from build123d import *
from build123d.topology import SkipClean

# Parameters (mm, degrees)
SKETCH2_R           = 2.5
BOSS_EXTRUDE1_DEPTH = 7
FILLET1_R           = 90
BOSS_EXTRUDE3_DEPTH = 15
SKETCH4_R           = 8
CUT_EXTRUDE1_DEPTH  = 10
BOSS_EXTRUDE4_START = 10
BOSS_EXTRUDE4_DEPTH = 10


with BuildPart() as part:
    # Sketch2 → Boss-Extrude1 (new body)
    with BuildSketch(Plane(origin=(0, 0, 0), x_dir=(1, 0, 0), z_dir=(0, 1, 0))):
        with BuildLine():
            Line((-4.24846021, -9.602113613), (13.572308451, -17.486922065))
            ThreePointArc((13.572308451, -17.486922065), (20.638500285, -15.805826469), (20.907079545, -8.547382103))
            Line((20.907079545, -8.547382103), (11.451696022, 4.891208687))
            ThreePointArc((11.451696022, 4.891208687), (9.270724445, 7.034926316), (6.472222222, 8.268031175))
            ThreePointArc((6.472222222, 8.268031175), (4.86754966, 9.30359932), (3.101845071, 10.031378627))
            Line((3.101845071, 10.031378627), (-8.821699821, 13.718308443))
            ThreePointArc((-8.821699821, 13.718308443), (-15.091857172, 11.987583677), (-16.147811194, 5.569231667))
            Line((-16.147811194, 5.569231667), (-12.308520784, -3.358124948))
            ThreePointArc((-12.308520784, -3.358124948), (-9.971976629, -6.504419403), (-6.472222222, -8.268031175))
            ThreePointArc((-6.472222222, -8.268031175), (-5.401685102, -9.003987898), (-4.24846021, -9.602113613))
        make_face()
        with Locations(Location((16, -12, 0), (0, 0, 270))):
            Circle(SKETCH2_R, mode=Mode.SUBTRACT)
        with Locations(Location((-10.604337088, 7.953252816, 0), (0, 0, 270))):
            Circle(SKETCH2_R, mode=Mode.SUBTRACT)
        with BuildLine():
            ThreePointArc((-4.694444444, -4.495797077), (0, -6.5), (4.694444444, -4.495797077))
            ThreePointArc((4.694444444, -4.495797077), (9, 0), (4.694444444, 4.495797077))
            ThreePointArc((4.694444444, 4.495797077), (0, 6.5), (-4.694444444, 4.495797077))
            ThreePointArc((-4.694444444, 4.495797077), (-9, 0), (-4.694444444, -4.495797077))
        make_face(mode=Mode.SUBTRACT)
    extrude(amount=BOSS_EXTRUDE1_DEPTH)

    # Fillet1
    fillet1_edges = [part.edges().sort_by_distance(p)[0] for p in [
        (6.472222222, 3.5, -8.268031175),
        (-6.472222222, 3.5, 8.268031175),
    ]]
    fillet(fillet1_edges, radius=FILLET1_R)

    # Sketch3 → Boss-Extrude3 (add)
    with BuildSketch(Plane(origin=(0, 7, 0), x_dir=(1, 0, 0), z_dir=(0, 1, 0))):
        with BuildLine():
            Line((-13.446880098, 1.012795393), (-12.308520784, -3.358124948))
            ThreePointArc((-12.308520784, -3.358124948), (-10.611843956, -5.907229762), (-8.121968415, -7.689690813))
            ThreePointArc((-8.121968415, -7.689690813), (-6.480430757, -8.483296944), (-4.855306799, -9.309994408))
            ThreePointArc((-4.855306799, -9.309994408), (-4.554226262, -9.460920841), (-4.24846021, -9.602113613))
            Line((-4.24846021, -9.602113613), (-1.454246479, -10.838414946))
            ThreePointArc((-1.454246479, -10.838414946), (10.979115699, -7.880432641), (11.451696022, 4.891208687))
            ThreePointArc((11.451696022, 4.891208687), (9.968863726, 6.507036925), (8.121968415, 7.689690813))
            ThreePointArc((8.121968415, 7.689690813), (6.480430757, 8.483296944), (4.855306799, 9.309994408))
            ThreePointArc((4.855306799, 9.309994408), (3.994892398, 9.710346787), (3.101845071, 10.031378627))
            Line((3.101845071, 10.031378627), (-3.895223267, 11.305534387))
            ThreePointArc((-3.895223267, 11.305534387), (-5.691953988, 10.727471116), (-6.207623157, 8.911848981))
            ThreePointArc((-6.207623157, 8.911848981), (-7.30582589, 4.892236012), (-11.232333003, 3.497288147))
            ThreePointArc((-11.232333003, 3.497288147), (-13.004436636, 2.847636589), (-13.446880098, 1.012795393))
        make_face()
        with BuildLine():
            ThreePointArc((4.694444444, -4.495797077), (9, 0), (4.694444444, 4.495797077))
            ThreePointArc((4.694444444, 4.495797077), (0, 6.5), (-4.694444444, 4.495797077))
            ThreePointArc((-4.694444444, 4.495797077), (-9, 0), (-4.694444444, -4.495797077))
            ThreePointArc((-4.694444444, -4.495797077), (0, -6.5), (4.694444444, -4.495797077))
        make_face(mode=Mode.SUBTRACT)
    extrude(amount=BOSS_EXTRUDE3_DEPTH)

    # Sketch4 → Cut-Extrude1 (cut)
    with BuildSketch(Plane(origin=(0, 22, 0), x_dir=(1, 0, 0), z_dir=(0, 1, 0))):
        Circle(SKETCH4_R)
    extrude(amount=-CUT_EXTRUDE1_DEPTH, mode=Mode.SUBTRACT)

    # Sketch5 → Boss-Extrude4 (add)
    with SkipClean():  # the faces are left unmerged after this step: merging them gives an invalid solid
        with BuildSketch(Plane(origin=(0, 12, 0), x_dir=(1, 0, 0), z_dir=(0, 1, 0)).offset(BOSS_EXTRUDE4_START)):
            with BuildLine():
                ThreePointArc((-7.111111111, 3.664982778), (-8, 0), (-7.111111111, -3.664982778))
                ThreePointArc((-7.111111111, -3.664982778), (-9, 0), (-7.111111111, 3.664982778))
            make_face()
            with BuildLine():
                ThreePointArc((7.111111111, -3.664982778), (9, 0), (7.111111111, 3.664982778))
                ThreePointArc((7.111111111, 3.664982778), (8, 0), (7.111111111, -3.664982778))
            make_face()
        extrude(amount=-BOSS_EXTRUDE4_DEPTH)


solid = part.part
Geometry: final body of the model. Coordinates: model frame, mm. A direction names the side the tool comes from. Coordinates: 2 decimals unless noted, no trailing zeros. Order: outer loops, then holes, each group sorted by start corner. A loop starts at its lowest first (then second) coordinate and runs counter-clockwise, first axis right, second up.
(1) Section query D-D (x = 12). Return the cut outline in (y, z).
(2) Section query A-A (z = -2). Return the cut outline in (x, y).
(3) Draft query along X for faces 1 (the face through (16.246, 3.451, 1.922)), 2 (the face through (20.57, 3.45, 15.89)), 3 (the face through (0.1, 5.9, -6.5)). Return one class per face: pulls with the +X half, pulls with the -X half, needs draft (parallel to the pull), parting line crosses it, or undercut.
(4) Section query B-B (y = 18). Return the cut outline in (x, z).
(5) Access query for faces 4 (the face through (0, 12, 7)), 5 (the face through (9, 6, 0)), 6 (the face through (3, 22, 8)), 7 (the face through (-12.886, 14.395, 1.142)), 8 (the face through (-0.35, 14.4, -10.66)). Directions: +Z, -Z, +X, -X, +Y, -Y. A direction counts if a zero-diameter tool reaches every point of the face in a straight line with its end or side. Return the directions, or none.
(6) Material intervals for probe 1 along Z at (x, y) = (-8.5, 2.5); probe 2 along Y at (x, z) = (-7, -6.5); probe 3 along Z at (x, y) = (-5, 12.5) (3 decimals), sorted ascending.
(7) First-contact query: pin 1 (3 mm diameter, centred on x = 0.5, z = 3.5, fed in from +Y); pin 2 (6.5 mm diameter, centred on x = 16, z = 12, fed in from +Y); pin 3 (6 mm diameter, centred on x = 7.5, y = 8, fed in from +Z); pin 4 (0.6 mm diameter, centred on x = -8, z = 1.5, fed in from -Y). Flat tips, straight axial feed; report the tip coordinate or a pass-through.
(8) Section query C-C (x = 16). Return the cut outline in (y, z), plus the area to 3 significant figures.
Solution:
1. outline: (0, -4.11) - (7, -4.11) - (7, -4.03) - (22, -4.03) - (22, 6.39) - (7, 6.39) - (7, 16.79) - (0, 16.79) - close
2. outline: (-14.61, 0) - (-8.53, 0) - (-8.53, 12) - (-7.75, 12) - (-7.75, 22) - (-13.45, 22) - (-13.45, 7) - (-14.61, 7) - close; (7.75, 12) - (8.53, 12) - (8.53, 0) - (13.49, 0) - (13.49, 7) - (12.88, 7) - (12.88, 22) - (7.75, 22) - close
3. face 1: pulls with the +X half
3. face 2: parting line crosses it
3. face 3: undercut
4. outline: (-13.45, -1.01) arc R2 ccw to (-11.23, -3.5) arc R4.5 cw to (-6.21, -8.91) arc R2 ccw to (-3.9, -11.31) - (3.1, -10.03) arc R10.5 ccw to (4.86, -9.31) arc R90 cw to (8.12, -7.69) arc R8.5 ccw to (11.45, -4.89) arc R10.56 ccw to (-1.45, 10.84) - (-4.25, 9.6) arc R10.5 ccw to (-4.86, 9.31) arc R90 cw to (-8.12, 7.69) arc R8.5 ccw to (-12.31, 3.36) - close; hole circle Ø16 at (0, 0)
5. face 4: +Y
5. face 5: -Y
5. face 6: +Z, -Z, +X, -X, +Y
5. face 7: +Z, -X, +Y
5. face 8: -Z, +X, +Y
6. probe 1: z = -13.62 to -9.3, -6.6 to -2.06, 2.06 to 7.5
6. probe 2: y = 0 to 7
6. probe 3: z = -11.193 to -6.245, 6.245 to 9.235
7. pin 1: passes through
7. pin 2: stops at y = 7
7. pin 3: stops at z = 16.05
7. pin 4: stops at y = 12
8. outline: (0, 1.57) - (7, 1.57) - (7, 9.5) - (0, 9.5) - close; (0, 14.5) - (7, 14.5) - (7, 18) - (0, 18) - close
8. area: 80.0 mm2
